The listing builds one solid part. Answer for the finished solid, in the listing's coordinates (mm). A direction names the side the tool comes from. Give positions to 0.01 mm unless a question says otherwise; leave off trailing zeros. Write each loop counter-clockwise with the first axis right and the second up, starting at its lowest first coordinate (ties: lowest second). Pieces come first, ordered by that corner, then holes. Notation, with made-up numbers: M 23.25,-30 L 71.25,-30 A29 cw 71.25,8 Z; hole C 85,32 d7. An arc over 180 degrees is marked long. Answer as a JSON object with one key per item and string values.
```python
from build123d import *

# Parameters (mm, degrees)
F0_R     = 31.75
F0_R_2   = 1.5748
F1_DEPTH = 6.35


with BuildPart() as f1:
    # F0 (on Top) → F1 (new body)
    with BuildSketch(Plane.XY):
        Circle(F0_R)
        with BuildLine():
            ThreePointArc((20.955, -19.427264), (-5.567411, -28.027389), (-26.789215, -9.943267))
            ThreePointArc((-26.789215, -9.943267), (-26.234197, -5.566779), (-22.324346, -3.523556))
            Line((-22.324346, -3.523556), (-6.638238, -3.523556))
            ThreePointArc((-6.638238, -3.523556), (-5.060266, -3.792571), (-3.66056, -4.569225))
            ThreePointArc((-3.66056, -4.569225), (5.8547, 0), (-3.66056, 4.569225))
            ThreePointArc((-3.66056, 4.569225), (-5.060266, 3.792571), (-6.638238, 3.523556))
            Line((-6.638238, 3.523556), (-22.324346, 3.523556))
            ThreePointArc((-22.324346, 3.523556), (-26.234197, 5.566779), (-26.789215, 9.943267))
            ThreePointArc((-26.789215, 9.943267), (-5.567411, 28.027389), (20.955, 19.427264))
            ThreePointArc((20.955, 19.427264), (21.896146, 17.928406), (22.225, 16.189387))
            Line((22.225, 16.189387), (22.225, 0))
            Line((22.225, 0), (22.225, -16.189387))
            ThreePointArc((22.225, -16.189387), (21.896146, -17.928406), (20.955, -19.427264))
        make_face(mode=Mode.SUBTRACT)
        Circle(F0_R_2, mode=Mode.SUBTRACT)
    extrude(amount=F1_DEPTH)


solid = f1.part
```
1. The mould has two halves that part along X. Classify faces 1 (the cylindrical face through (-1.25, -0.96, 3.13)), 2 (the cylindrical face through (-6.883, -30.995, 3.131)), 3 (the flat face through (-14, 3.524, 3)), 4 (the flat face through (0, 3, 6.35)): released by +X, released by -X, zero draft, split by the parting line, or undercut.
Verdict:
{"face 1": "undercut", "face 2": "split by the parting line", "face 3": "undercut", "face 4": "zero draft"}
2. A cutting plane is placed at D-D, the plane y = 7. Give the vertices of the cut face in (x, z) (3 decimals), plus the area to 3 significant figures.
Verdict:
{"outline": "M -30.969,0 L -26.91,0 L -26.91,6.35 L -30.969,6.35 Z; M 22.225,0 L 30.969,0 L 30.969,6.35 L 22.225,6.35 Z", "area": "81.3 mm2"}
3. A cutting plane is placed at A-A, the plane z = 5.5. Count the separate pieces of the cut face and the enclosed holes in it, plus the area to 3 significant figures.
Verdict:
{"separate pieces": "1", "enclosed holes": "2", "area": "1,040 mm2"}
4. A cutting plane is placed at B-B, the plane y = 0. Give the vertices of the cut face in (x, z) (3 decimals), plus the area to 3 significant figures.
Verdict:
{"outline": "M -31.75,0 L -1.575,0 L -1.575,6.35 L -31.75,6.35 Z; M 1.575,0 L 5.855,0 L 5.855,6.35 L 1.575,6.35 Z; M 22.225,0 L 31.75,0 L 31.75,6.35 L 22.225,6.35 Z", "area": "279 mm2"}
5. For faces 5 (the cylindrical face through (-5.04, 3.8, 3.13)), 6 (the flat face through (0, 3, 0)), determine the directions among +Z, -Z, +X, -X, +Y, -Y from which every point of the face is accessible in a straight line to the end or side of a thin tool.
Verdict:
{"face 5": "+Z, -Z", "face 6": "-Z, +X, -X, +Y, -Y"}
6. Consider line 1 along Y through (x, z) = (0, 4.75) (3 decimals); line 2 along Y through (x, z) = (-2, 6); line 3 along Y through (x, z) = (-26, 2). Determine where each line is inside the solid, lowest interval first.
Verdict:
{"line 1": "y = -31.75 to -28.575, -5.855 to -1.575, 1.575 to 5.855, 28.575 to 31.75", "line 2": "y = -31.69 to -28.5, -5.5 to 5.5, 28.5 to 31.69", "line 3": "y = -18.22 to -11.85, -5.26 to 5.26, 11.85 to 18.22"}
7. A cutting plane is placed at C-C, the plane x = 0. Give the vertices of the cut face in (y, z) (3 decimals).
Verdict:
{"outline": "M -31.75,0 L -28.575,0 L -28.575,6.35 L -31.75,6.35 Z; M -5.855,0 L -1.575,0 L -1.575,6.35 L -5.855,6.35 Z; M 1.575,0 L 5.855,0 L 5.855,6.35 L 1.575,6.35 Z; M 28.575,0 L 31.75,0 L 31.75,6.35 L 28.575,6.35 Z"}
8. Flat-ended cylindrical pins translate along their axes: pin 1 (3 mm diameter, centred on x = -13.5, z = 4, fed in from -Y); pin 2 (3 mm diameter, centred on x = 0, y = 0, fed in from -Z); pin 3 (1.5 mm diameter, centred on x = 0.5, z = 2.5, fed in from +Y); pin 4 (2 mm diameter, centred on x = -25, z = 1.5, fed in from -Y). Find the tip coordinate at first contact, or state that the pin passes through.
Verdict:
{"pin 1": "stops at y = -29.39", "pin 2": "passes through", "pin 3": "stops at y = 31.75", "pin 4": "stops at y = -20.79"}
